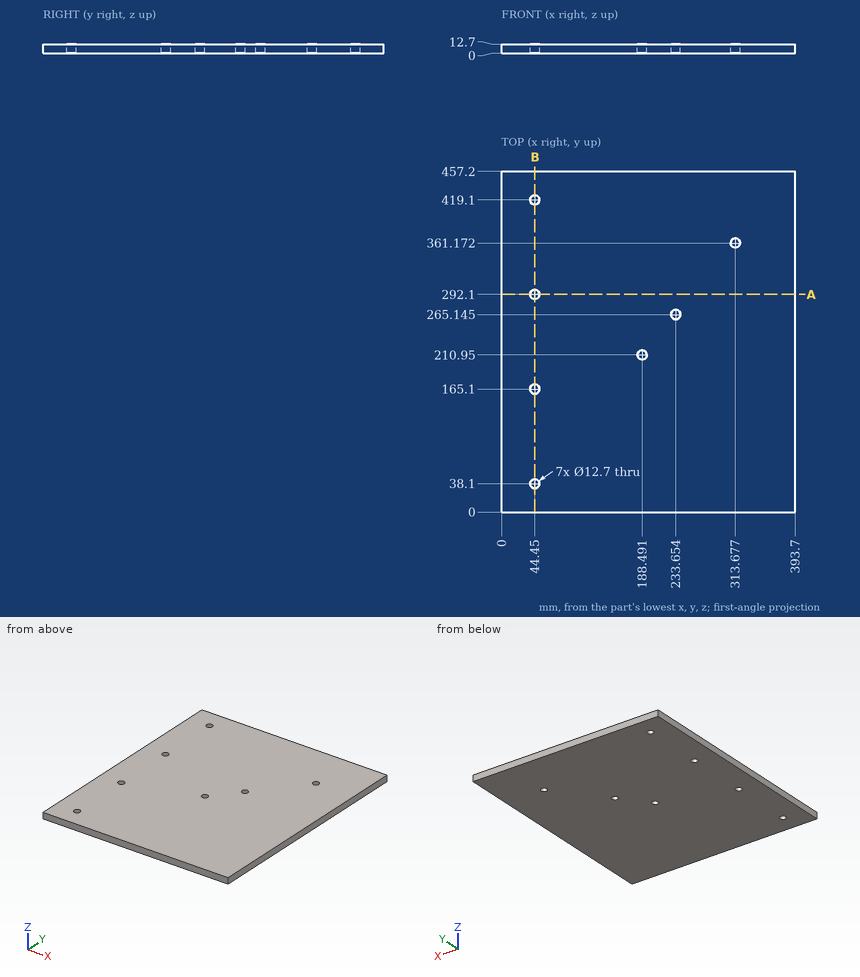
Here's the drawing with two shaded views (mm, measured from the low corner). I have some questions. Give positions to 0.01 mm unless a question says otherwise; leave off trailing zeros. Order: outer loops, then holes, each group sorted by start corner. A loop starts at its lowest first (then second) coordinate and runs counter-clockwise, first axis right, second up.
Q1. If I drill on line 1 along X through (y, z) = (37, 5.5) (1 decimal); line 2 along X through (y, z) = (365.5, 3.25) (1 decimal), over which ranges is the centre line in solid material (lowest first)?
Q2. Suppose I cut it at B-B, the plane x = 44.45. Write out the boundary of the cut face in (y, z).
Q3. Suppose I cut it at A-A, the plane y = 292.1. Write out the boundary of the cut face in (x, z), and give its area (3 significant figures).
Solution:
1. line 1: x = 0 to 38.2, 50.7 to 393.7
1. line 2: x = 0 to 309, 318.3 to 393.7
2. outline: (0, 0) - (31.75, 0) - (31.75, 12.7) - (0, 12.7) - close; (44.45, 0) - (158.75, 0) - (158.75, 12.7) - (44.45, 12.7) - close; (171.45, 0) - (285.75, 0) - (285.75, 12.7) - (171.45, 12.7) - close; (298.45, 0) - (412.75, 0) - (412.75, 12.7) - (298.45, 12.7) - close; (425.45, 0) - (457.2, 0) - (457.2, 12.7) - (425.45, 12.7) - close
3. outline: (0, 0) - (38.1, 0) - (38.1, 12.7) - (0, 12.7) - close; (50.8, 0) - (393.7, 0) - (393.7, 12.7) - (50.8, 12.7) - close
3. area: 4,840 mm2
